The listing builds one solid part. Answer for the finished solid, in the listing's coordinates (mm). Coordinates: 2 decimals unless noted, no trailing zeros. Write each loop counter-clockwise with the first axis right and the second up, starting at its lowest first coordinate (ties: lowest second). Pieces come first, ordered by that corner, then holes.
```python
from build123d import *

# Parameters (mm, degrees)
EXTRUDE_2_DEPTH = 1


with BuildPart() as part:
    # Sketch 2 → Extrude 2 (new, symmetric)
    with BuildSketch(Plane.XY):
        Polygon((-75, 40), (75, 40), (75, -40), (-75, -40), (-95, 0), align=None)
    extrude(amount=EXTRUDE_2_DEPTH, both=True)

    # Sketch 2_5 → Revolve 5 (revolve)
    with BuildSketch(Plane.XY, mode=Mode.PRIVATE) as revolve_5_sk:
        Polygon((-85, 0), (-98.554984954, 30), (-98.554984954, 0), align=None)
    revolve(revolve_5_sk.sketch.rotate(Axis((-1003.811687892, 0, 0), (1, 0, 0)), 90), axis=Axis((-1003.811687892, 0, 0), (1, 0, 0)))


solid = part.part
```
(1) Find the intervals of material crossed by probe 1 along Z at (x, y) = (28, 23); probe 2 along Y at (x, z) = (-80, 0.5); probe 3 along X at (y, z) = (-12.5, 23), in increasing order.
(2) Section A-A, the plane x = 13 is taken. Write down the section's boundary in (y, z), plus the area to 3 significant figures.
(3) Section B-B, the plane y = 0 is taken. Write down the section's boundary in (x, z), plus the area to 3 significant figures.
(4) Each of these flat-tipped pins is pushed along its axis until it touches: pin 1 (4 mm diameter, centred on x = 11, y = -7, fed in from +Z); pin 2 (1 mm diameter, centred on y = 19.5, z = 2.5, fed in from +X); pin 3 (6 mm diameter, centred on x = -47, y = -22, fed in from -Z). Where does it stop, or does it pass through?
(5) Section C-C, the plane x = -80.5 is taken. Write down the section's boundary in (y, z).
(6) For a pull along X with two mould halves and no side action, classify faces 1 (the flat face through (-6, 1, -1)), 2 (the flat face through (-98.555, 0, 0)), 3 (the flat face through (-82.3, -25.4, 0)), 4 (the flat face through (-82.5, 25, 0)) as pulls with the +X half, pulls with the -X half, needs draft (parallel to the pull), parting line crosses it, or undercut.
Solution:
1. probe 1: z = -1 to 1
1. probe 2: y = -30 to 30
1. probe 3: x = -98.55 to -96.83
2. outline: (-40, -1) - (40, -1) - (40, 1) - (-40, 1) - close
2. area: 160 mm2
3. outline: (-98.55, -30) - (-85.45, -1) - (75, -1) - (75, 1) - (-85.45, 1) - (-98.55, 30) - close
3. area: 727 mm2
4. pin 1: stops at z = 1
4. pin 2: stops at x = -93.66
4. pin 3: stops at z = -1
5. outline: (-29, -1) - (29, -1) - (29, 1) - (-29, 1) - close
6. face 1: needs draft
6. face 2: pulls with the -X half
6. face 3: undercut
6. face 4: undercut
